Input: part model. Units: mm. Frame: model coordinates. Coordinates: 2 decimals unless noted, no trailing zeros. Write each loop counter-clockwise with the first axis right and the second up, starting at its lowest first coordinate (ties: lowest second). Pieces come first, ordered by that corner, then holes. Notation, with made-up numbers: M 79.25,53 L 105.25,53 A9 ccw 105.25,66 Z; hole C -35,-32.75 d2. An arc over 180 degrees is marked long. Write each question's results on one line, items separated by ' | '. Start each with the question number.
1. Section query C-C, the plane x = -38.5. Output: boundary loops of the cut face in (y, z), and give its area (3 significant figures).
2. Section query D-D, the plane z = 28. Output: boundary loops of the cut face in (x, y).
3. Section query B-B, the plane y = 0. Output: boundary loops of the cut face in (x, z), and give its area (3 significant figures).
4. Section query A-A, the plane x = 12.7. Output: boundary loops of the cut face in (y, z), and give its area (3 significant figures).
5. Ray query, probe 1 along Y at (x, z) = (-12.7, -26.5); probe 2 along Z at (x, y) = (44, 33); probe 3 along Y at (x, z) = (12, -38). Return the intervals inside material, ascending.
6. First-contact query: pin 1 (3 mm diameter, centred on x = -13.5, y = -2, fed in from -Z). Flat tip, straight axial feed; report the tip coordinate or a pass-through.
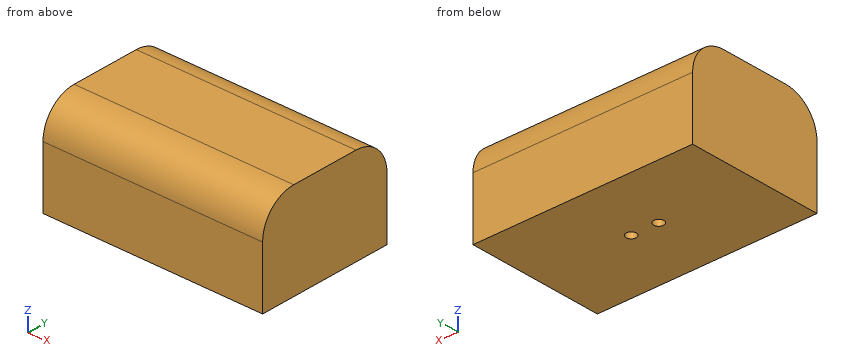
```python
from build123d import *

# Parameters (mm, degrees)
SKETCH1_W           = 203.2
SKETCH1_H           = 127
BOSS_EXTRUDE1_DEPTH = 44.45
FILLET1_R           = 31.75
SKETCH3_R           = 4.7625
CUT_EXTRUDE1_DEPTH  = 25.4


with BuildPart() as part:
    # Sketch1 → Boss-Extrude1 (new, symmetric)
    with BuildSketch(Plane.XY):
        Rectangle(SKETCH1_W, SKETCH1_H)
    extrude(amount=BOSS_EXTRUDE1_DEPTH, both=True)

    # Fillet1
    fillet1_edges = [part.edges().sort_by_distance(p)[0] for p in [
        (0, -63.5, 44.45),
        (0, 63.5, 44.45),
    ]]
    fillet(fillet1_edges, radius=FILLET1_R)

    # Sketch3 → Cut-Extrude1 (cut)
    with BuildSketch(Plane(origin=(0, 0, -44.45), x_dir=(-1, 0, 0), z_dir=(0, 0, -1))):
        with Locations((-12.7, 0)):
            Circle(SKETCH3_R)
        with Locations((12.7, 0)):
            Circle(SKETCH3_R)
    extrude(amount=-CUT_EXTRUDE1_DEPTH, mode=Mode.SUBTRACT)


solid = part.part
```
Answer:
1) outline: M -63.5,-44.45 L 63.5,-44.45 L 63.5,12.7 A31.75 ccw 31.75,44.45 L -31.75,44.45 A31.75 ccw -63.5,12.7 Z | area: 10,900 mm^2
2) outline: M -101.6,-59.57 L 101.6,-59.57 L 101.6,59.57 L -101.6,59.57 Z
3) outline: M -101.6,-44.45 L -17.46,-44.45 L -17.46,-19.05 L -7.94,-19.05 L -7.94,-44.45 L 7.94,-44.45 L 7.94,-19.05 L 17.46,-19.05 L 17.46,-44.45 L 101.6,-44.45 L 101.6,44.45 L -101.6,44.45 Z | area: 17,600 mm^2
4) outline: M -63.5,-44.45 L -4.76,-44.45 L -4.76,-19.05 L 4.76,-19.05 L 4.76,-44.45 L 63.5,-44.45 L 63.5,12.7 A31.75 ccw 31.75,44.45 L -31.75,44.45 A31.75 ccw -63.5,12.7 Z | area: 10,600 mm^2
5) probe 1: -63.5 to -4.76, 4.76 to 63.5 | probe 2: -44.45 to 44.43 | probe 3: -63.5 to -4.71, 4.71 to 63.5
6) pin 1: z = -19.05
